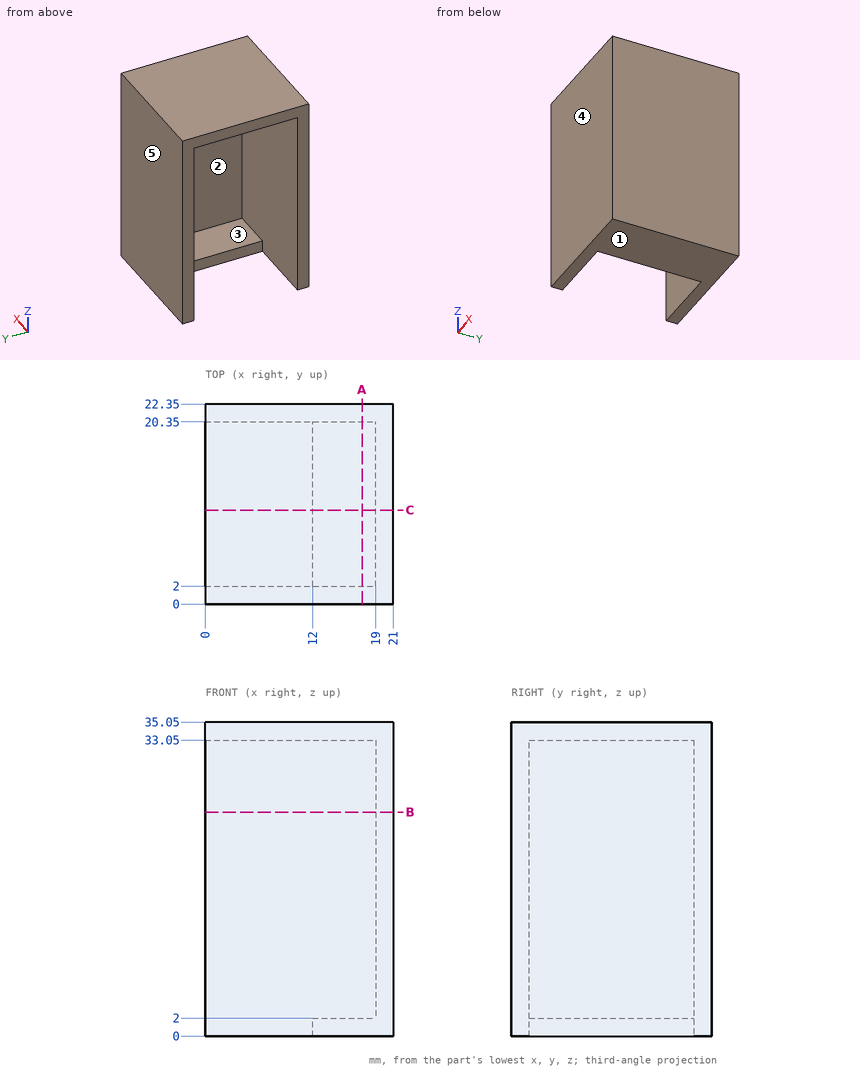
Job drawing, mm, ordinate dimensions from the low corner. One solid piece. A direction names the side the tool comes from. Coordinates: 2 decimals unless noted, no trailing zeros. Write each loop counter-clockwise with the first axis right and the second up, starting at its lowest first coordinate (ties: lowest second). Pieces come first, ordered by that corner, then holes. Notation, with made-up numbers: (22.5, -31.75) - (81.5, -31.75) arc R27 cw to (81.5, -15.75) - close; hole circle Ø2 at (-39, -31.75). An arc over 180 degrees is marked (long way). Use a Markdown table: item, result. Add a question column.
Item 1: Band-saw the part on A-A, the plane x = 17.5. Give the cut face in (y, z).
Item 2: 3-axis set-ups, long thin cutter, end or side, ignore diameter. For the marked faces 1 and 2: which of +Z, -Z, +X, -X, +Y, -Y reach the whole face in a straight line?
Item 3: Mould opens along Y. For the marked faces 3, 4 and 5 say: pulls with the +Y half, pulls with the -Y half, needs draft (parallel to the pull), parting line crosses it, or undercut.
Item 4: Band-saw the part on B-B, the plane z = 25. Give the cut face in (x, y), and give its area (3 significant figures).
Item 5: Drill centre lines: L1, parallel to Y at x = 10, z = 25; L2, parallel to Z at x = 18.25, y = 6.75; L3, parallel to X at y = 15.25, z = 30.5. Where is each one in solid material? Low to high. Write a range as from..to.
Item 6: Band-saw the part on C-C, the plane y = 10.5. Give the cut face in (x, z).
Item 7: Flat gauge pins, fed straight in: pin 1 (2 mm diameter, centred on y = 11.5, z = 5, fed in from -X); pin 2 (2 mm diameter, centred on y = 15, z = 1, fed in from -X); pin 3 (5.5 mm diameter, centred on x = 7.5, y = 15.5, fed in from -Z). Where does each tip first touch, or does it go through?
Numbers:
| question | item | result |
|---|---|---|
| 1 | outline | (0, 0) - (22.35, 0) - (22.35, 35.05) - (0, 35.05) - close; hole (2, 2) - (20.35, 2) - (20.35, 33.05) - (2, 33.05) - close |
| 2 | face 1 | -Z, +X, -X, +Y, -Y |
| 2 | face 2 | -X |
| 3 | face 3 | undercut |
| 3 | face 4 | pulls with the -Y half |
| 3 | face 5 | pulls with the +Y half |
| 4 | outline | (0, 0) - (21, 0) - (21, 22.35) - (0, 22.35) - (0, 20.35) - (19, 20.35) - (19, 2) - (0, 2) - close |
| 4 | area | 121 mm2 |
| 5 | L1 | 0..2, 20.35..22.35 |
| 5 | L2 | 0..2, 33.05..35.05 |
| 5 | L3 | 19..21 |
| 6 | outline | (0, 33.05) - (19, 33.05) - (19, 2) - (12, 2) - (12, 0) - (21, 0) - (21, 35.05) - (0, 35.05) - close |
| 7 | pin 1 | x = 19 |
| 7 | pin 2 | x = 12 |
| 7 | pin 3 | z = 33.05 |
